```python
from build123d import *

# Parameters (mm, degrees)
SKETCH1_R           = 12.5
BOSS_EXTRUDE1_DEPTH = 7.5
SKETCH2_W           = 35
SKETCH2_H           = 8.580767914
BOSS_EXTRUDE2_DEPTH = 25
SKETCH3_W           = 25
SKETCH3_H           = 8.580767914
CUT_EXTRUDE1_DEPTH  = 20
SKETCH4_R           = 2.5
BOSS_EXTRUDE3_DEPTH = 5
SKETCH5_R           = 2.5
BOSS_EXTRUDE4_DEPTH = 5
CHAMFER1_SIZE       = 5
CHAMFER2_SIZE       = 5
FILLET1_R           = 2.5
FILLET2_R           = 2.5


with BuildPart() as part:
    # Sketch1 → Boss-Extrude1 (new body)
    with BuildSketch(Plane(origin=(0, 0, 0), x_dir=(1, 0, 0), z_dir=(0, 1, 0))):
        Circle(SKETCH1_R)
    extrude(amount=BOSS_EXTRUDE1_DEPTH)

    # Sketch2 → Boss-Extrude2 (add)
    with BuildSketch(Plane(origin=(0, 7.5, 0), x_dir=(1, 0, 0), z_dir=(0, 1, 0))):
        Rectangle(SKETCH2_W, SKETCH2_H)
    extrude(amount=BOSS_EXTRUDE2_DEPTH)

    # Sketch3 → Cut-Extrude1 (cut)
    with BuildSketch(Plane(origin=(0, 32.5, 0), x_dir=(1, 0, 0), z_dir=(0, 1, 0))):
        Rectangle(SKETCH3_W, SKETCH3_H)
    extrude(amount=-CUT_EXTRUDE1_DEPTH, mode=Mode.SUBTRACT)

    # Sketch4 → Boss-Extrude3 (add)
    with BuildSketch(Plane(origin=(-12.5, 0, 0), x_dir=(0, 0, -1), z_dir=(1, 0, 0))):
        with Locations((0, 27.5)):
            Circle(SKETCH4_R)
    extrude(amount=BOSS_EXTRUDE3_DEPTH)

    # Sketch5 → Boss-Extrude4 (add)
    with BuildSketch(Plane.ZY.offset(-12.5)):
        with Locations((0, 27.5)):
            Circle(SKETCH5_R)
    extrude(amount=BOSS_EXTRUDE4_DEPTH)

    # Chamfer1
    chamfer1_edges = [part.edges().sort_by_distance(p)[0] for p in [
        (-12.5, 12.5, 0),
    ]]
    chamfer(chamfer1_edges, length=CHAMFER1_SIZE)

    # Chamfer2
    chamfer2_edges = [part.edges().sort_by_distance(p)[0] for p in [
        (12.5, 12.5, 0),
    ]]
    chamfer(chamfer2_edges, length=CHAMFER2_SIZE)

    # Fillet1
    fillet1_edges = [part.edges().sort_by_distance(p)[0] for p in [
        (-7.5, 27.5, 2.5),
    ]]
    fillet(fillet1_edges, radius=FILLET1_R)

    # Fillet2
    fillet2_edges = [part.edges().sort_by_distance(p)[0] for p in [
        (7.5, 27.5, -2.5),
    ]]
    fillet(fillet2_edges, radius=FILLET2_R)


solid = part.part
```
The listing builds one solid part. Answer for the finished solid, in the listing's coordinates (mm). A direction names the side the tool comes from. Round coordinates to 2 decimals unless told otherwise and drop trailing zeros. Write each loop counter-clockwise with the first axis right and the second up, starting at its lowest first coordinate (ties: lowest second). Pieces come first, ordered by that corner, then holes. Notation, with made-up numbers: (29.5, 53) -> (39.5, 53) arc R36 ccw to (39.5, 90) -> close; hole circle Ø4 at (-6, -2.5). An arc over 180 degrees is marked (long way). Answer as a JSON object with one key per item and string values. Group by question number.
Q1. Determine the mould class of faces 6 (the face through (15, 32.5, 0)), 7 (the face through (-10, 15, 0)), 8 (the face through (-17.5, 20, 0)) for opening direction X: pulls with the +X half, pulls with the -X half, needs draft (parallel to the pull), parting line crosses it, or undercut.
Q2. Straight lines are drawn through the part: line 1 along X through (y, z) = (19, -0.75); line 2 along Y through (x, z) = (-7, -9.5); line 3 along Y through (x, z) = (9, 0). For each, find the intervals that lie inside material, in ascending order.
Q3. Which of the six approach directions +Z, -Z, +X, -X, +Y, -Y give full straight-line access (tool end or side, diameter ignored) to faces 1 (the face through (-11, 30, 0)), 2 (the face through (0, 7.5, -8)), 3 (the face through (0, 12.5, 0)), 4 (the face through (0, 7.5, 7)), 5 (the face through (10, 15, 0))?
Q4. Section B-B (x = 0) is taken. Write down the section's boundary in (y, z), plus the area to 3 significant figures.
Q5. Section A-A (y = 27.5) is taken. Write down the section's boundary in (x, z), plus the area to 3 significant figures.
Q6. Section C-C (z = 0) is taken. Write down the section's boundary in (x, y), plus the area to 3 significant figures.
Q7. Each of these flat-tipped pins is pushed along its axis until it touches: pin 1 Ø8 at (y, z) = (7, 9.5) entering from +X (3 decimals); pin 2 Ø4.5 at (x, z) = (-13.5, 2) entering from -Y; pin 3 Ø2.5 at (x, z) = (3.5, 10) entering from +Y; pin 4 Ø8 at (x, y) = (11.5, 15.5) entering from -Z. Where does it stop, or does it pass through?
Q8. Section D-D (x = -8) is taken. Write down the section's boundary in (y, z).
Check values:
{
 "1": {"face 6": "needs draft", "face 7": "undercut", "face 8": "pulls with the -X half"},
 "2": {"line 1": "-17.5 to -12.5, 12.5 to 17.5", "line 2": "0 to 7.5", "line 3": "0 to 14, 25.21 to 29.79"},
 "3": {"face 1": "none", "face 2": "-Z, +X, -X, +Y", "face 3": "+Z, -Z, +Y", "face 4": "+Z, +X, -X, +Y", "face 5": "+Z, -Z"},
 "4": {"outline": "(0, -12.5) -> (7.5, -12.5) -> (7.5, -4.29) -> (12.5, -4.29) -> (12.5, 4.29) -> (7.5, 4.29) -> (7.5, 12.5) -> (0, 12.5) -> close", "area": "230 mm^2"},
 "5": {"outline": "(-17.5, -4.29) -> (-12.5, -4.29) -> (-12.5, -2.5) -> (-10, -2.5) arc R2.5 ccw to (-10, 2.5) -> (-12.5, 2.5) -> (-12.5, 4.29) -> (-17.5, 4.29) -> close; (10, -2.5) -> (12.5, -2.5) -> (12.5, -4.29) -> (17.5, -4.29) -> (17.5, 4.29) -> (12.5, 4.29) -> (12.5, 2.5) -> (10, 2.5) arc R2.5 ccw to start", "area": "130 mm^2"},
 "6": {"outline": "(-17.5, 7.5) -> (-12.5, 7.5) -> (-12.5, 0) -> (12.5, 0) -> (12.5, 7.5) -> (17.5, 7.5) -> (17.5, 32.5) -> (12.5, 32.5) -> (12.5, 30) -> (10, 30) arc R2.5 ccw to (10, 25) -> (12.5, 25) -> (12.5, 17.5) -> (7.5, 12.5) -> (-7.5, 12.5) -> (-12.5, 17.5) -> (-12.5, 25) -> (-10, 25) arc R2.5 ccw to (-10, 30) -> (-12.5, 30) -> (-12.5, 32.5) -> (-17.5, 32.5) -> close", "area": "632 mm^2"},
 "7": {"pin 1": "x = 11.225", "pin 2": "y = 0", "pin 3": "y = 7.5", "pin 4": "z = -4.29"},
 "8": {"outline": "(0, -9.6) -> (7.5, -9.6) -> (7.5, -4.29) -> (13, -4.29) -> (13, 4.29) -> (7.5, 4.29) -> (7.5, 9.6) -> (0, 9.6) -> close; circle Ø3 at (27.5, 0)"}
}
